```python
from build123d import *

# Parameters (mm, degrees)
CHAMFER1_SIZE = 0.2
FILLET1_R     = 0.3


with BuildPart() as part:
    # Sketch1 → Revolve1 (revolve)
    with BuildSketch(Plane(origin=(0, 0, 0), x_dir=(0, 0, -1), z_dir=(1, 0, 0)), mode=Mode.PRIVATE) as revolve1_sk:
        Polygon((-2, 2.5), (2, 2.5), (2, 5.8), (1.2, 5.8), (1.2, 5), (-2, 5), align=None)
    revolve(revolve1_sk.sketch.rotate(Axis((0, 0, 0), (0, 0, -1)), 90), axis=Axis((0, 0, 0), (0, 0, -1)))

    # Chamfer1
    chamfer1_edges = [part.edges().sort_by_distance(p)[0] for p in [
        (-5, 0, 2),
        (-2.5, 0, -2),
        (-2.5, 0, 2),
    ]]
    chamfer(chamfer1_edges, length=CHAMFER1_SIZE)

    # Sketch2 → Cut-Revolve1 (revolve, cut)
    with BuildSketch(Plane(origin=(0, 0, 0), x_dir=(0, 0, -1), z_dir=(1, 0, 0)), mode=Mode.PRIVATE) as cut_revolve1_sk:
        Polygon((-2, 4.317089392), (-1.556756286, 4.317089392), (-1.556756286, 4.186077714), (-2, 4.186077714), (-2, 3.134478417), (-1.668024824, 3.134478417), (-1.668024824, 3.005528354), (-2, 3.005528354), (-2, 2.264675566), (-2.552130355, 2.264675566), (-2.552130355, 4.329651261), (-2, 4.329651261), align=None)
    cut_revolve1 = revolve(cut_revolve1_sk.sketch.rotate(Axis((0, 0, -2), (0, 0, 1)), 90), axis=Axis((0, 0, -2), (0, 0, 1)), mode=Mode.SUBTRACT)

    # Mirror3: Cut-Revolve1 across plane
    add(cut_revolve1.mirror(Plane.XY), mode=Mode.SUBTRACT)

    # Fillet1
    fillet1_edges = [part.edges().sort_by_distance(p)[0] for p in [
        (4.186077714, 0, 2),
        (4.186077714, 0, -2),
    ]]
    fillet(fillet1_edges, radius=FILLET1_R)


solid = part.part
```
Work out the finished part from the listing and answer in its coordinate system (mm). A direction names the side the tool comes from. Give positions to 0.01 mm unless a question says otherwise; leave off trailing zeros. Loops run counter-clockwise (first coordinate to the right, second up) from the corner with the lowest first, then second, coordinate; pieces in that order, holes last. Notation, with made-up numbers: (77.25, 25.5) -> (111.25, 25.5) arc R21 ccw to (111.25, 50.5) -> close; hole circle Ø4 at (-27, -35). An arc over 180 degrees is marked (long way). Write item = value, one per line. Start each with the question number.
(1) Find the intervals of material crossed by probe 1 along Y at (x, z) = (0, -0.3); probe 2 along Z at (x, y) = (3.75, 4.25); probe 3 along X at (y, z) = (-2.25, -0.65), in increasing order. Write a range as from..to.
(2) Which of the six approach directions +Z, -Z, +X, -X, +Y, -Y give full straight-line access (tool end or side, diameter ignored) to faces 1 (the flat face through (2, -5, -1.2)), 2 (the flat face through (3, -2, 2))?
(3) Given pin 1 Ø1.9 at (x, y) = (-0.5, -1.5) entering from -Z; pin 2 Ø4.5 at (x, y) = (0, 0) entering from +Z; pin 3 Ø2 at (x, z) = (-3, 0.5) entering from +Y, each flat-ended and moving along its own axis, determine where each tip first touches the part or whether it passes through.
(4) The mould has two halves that part along Y. Classify faces 3 (the cylindrical face through (-5, 0, 0)), 4 (the cylindrical face through (-2.5, -0.1, 0)), 5 (the flat face through (4, 2, -2)): +Y half, -Y half, draft (parallel to the pull), parting line (faces both ways), or undercut.
(5) Find section B-B on x = 5.25. Give the vertices of the cut face in (y, z), and give its area (3 significant figures).
(6) Find section A-A on z = -0.2. Give the vertices of the cut face in (x, y).
From the geometry:
q1.probe_1 = -5..-2.5, 2.5..5
q1.probe_2 = -2..-1.2
q1.probe_3 = -4.47..-1.09, 1.09..4.47
q2.face_1 = +Z
q2.face_2 = +Z, +X, -X, +Y, -Y
q3.pin_1 = -1.83
q3.pin_2 = through
q3.pin_3 = 4.58
q4.face_3 = parting line
q4.face_4 = undercut
q4.face_5 = draft
q5.outline = (-2.47, -2) -> (2.47, -2) -> (2.47, -1.2) -> (-2.47, -1.2) -> close
q5.area = 3.94 mm^2
q6.outline = circle Ø10 at (0, 0); hole circle Ø5 at (0, 0)
